The listing builds one solid part. Answer for the finished solid, in the listing's coordinates (mm). A direction names the side the tool comes from. Give positions to 0.01 mm unless a question says otherwise; leave off trailing zeros. Order: outer loops, then holes, each group sorted by start corner. A loop starts at its lowest first (then second) coordinate and runs counter-clockwise, first axis right, second up. Notation, with made-up numbers: (71, 51.25) - (93, 51.25) arc R27 cw to (93, 69.25) - close; hole circle Ø8 at (-39.5, 14.25). An arc over 180 degrees is marked (long way). Answer in a Markdown table with one row per item. Add a question column.
```python
from build123d import *

# Parameters (mm, degrees)
SKETCH1_R           = 8
BOSS_EXTRUDE1_DEPTH = 6.3
SKETCH2_R           = 3.5
BOSS_EXTRUDE2_DEPTH = 7.5
SKETCH3_R           = 3
CUT_EXTRUDE1_DEPTH  = 7.5
SKETCH5_W           = 1.3
SKETCH5_H           = 2.5
BOSS_EXTRUDE3_DEPTH = 0.3


with BuildPart() as part:
    # Sketch1 → Boss-Extrude1 (new body)
    with BuildSketch(Plane.XY):
        Circle(SKETCH1_R)
    extrude(amount=BOSS_EXTRUDE1_DEPTH)

    # Sketch2 → Boss-Extrude2 (add)
    with BuildSketch(Plane.XY.offset(6.3)):
        Circle(SKETCH2_R)
    extrude(amount=BOSS_EXTRUDE2_DEPTH)

    # Sketch3 → Cut-Extrude1 (cut)
    with BuildSketch(Plane.XY.offset(13.8)):
        Circle(SKETCH3_R)
    extrude(amount=-CUT_EXTRUDE1_DEPTH, mode=Mode.SUBTRACT)

    # Sketch5 → Boss-Extrude3 (add)
    with BuildSketch(Plane.XY.offset(6.3)):
        with Locations((-7.3, 0)):
            Rectangle(SKETCH5_W, SKETCH5_H)
    extrude(amount=BOSS_EXTRUDE3_DEPTH)


solid = part.part
```
(1) Find section D-D, the plane z = 3.25. Write down the section's boundary in (x, y), plus the area to 3 significant figures.
(2) Find section A-A, the plane y = 0. Write down the section's boundary in (x, z).
(3) Find section C-C, the plane z = 10. Write down the section's boundary in (x, y).
(4) Straight lines are drawn through the part: line 1 (Y direction, x = 0, z = 10.75); line 2 (Z direction, x = 3.5, y = 6.5); line 3 (Y direction, x = -2.75, z = 9.25). For each, find the intervals that lie inside material, in ascending order.
(5) The mould has two halves that part along X. Classify faces 1 (the face through (-3, 0, 10)), 2 (the face through (-1.73, -7.81, 3.11)), 3 (the face through (-7, 0, 6.6)): +X half, -X half, draft (parallel to the pull), parting line (faces both ways), or undercut.
(6) Find section B-B, the plane x = 0. Write down the section's boundary in (y, z), plus the area to 3 significant figures.
(7) Each of these flat-tipped pins is pushed along its axis until it touches: P1, Ø6, axis at y = 3, z = 7.5, coming from the -X side; P2, Ø4, axis at x = -5, z = 5.5, coming from the -Y side; P3, Ø1, axis at x = 1.5, z = 2, coming from the -Y side. Where does it stop, or does it pass through?
(8) For faces 4 (the face through (0, 0, 0)), 5 (the face through (3.233, -1.341, 9.997)), determine the directions among +Z, -Z, +X, -X, +Y, -Y from which every point of the face is accessible in a straight line to the end or side of a thin tool.
Answer key:
| question | item | result |
|---|---|---|
| 1 | outline | circle Ø16 at (0, 0) |
| 1 | area | 201 mm² |
| 2 | outline | (-8, 0) - (8, 0) - (8, 6.3) - (3.5, 6.3) - (3.5, 13.8) - (3, 13.8) - (3, 6.3) - (-3, 6.3) - (-3, 13.8) - (-3.5, 13.8) - (-3.5, 6.3) - (-6.65, 6.3) - (-6.65, 6.6) - (-7.95, 6.6) - (-7.95, 6.3) - (-8, 6.3) - close |
| 3 | outline | circle Ø7 at (0, 0); hole circle Ø6 at (0, 0) |
| 4 | line 1 | -3.5 to -3, 3 to 3.5 |
| 4 | line 2 | 0 to 6.3 |
| 4 | line 3 | -2.17 to -1.2, 1.2 to 2.17 |
| 5 | face 1 | undercut |
| 5 | face 2 | parting line |
| 5 | face 3 | draft |
| 6 | outline | (-8, 0) - (8, 0) - (8, 6.3) - (3.5, 6.3) - (3.5, 13.8) - (3, 13.8) - (3, 6.3) - (-3, 6.3) - (-3, 13.8) - (-3.5, 13.8) - (-3.5, 6.3) - (-8, 6.3) - close |
| 6 | area | 108 mm² |
| 7 | P1 | x = -8 |
| 7 | P2 | y = -7.42 |
| 7 | P3 | y = -7.94 |
| 8 | face 4 | -Z, +X, -X, +Y, -Y |
| 8 | face 5 | +Z |
